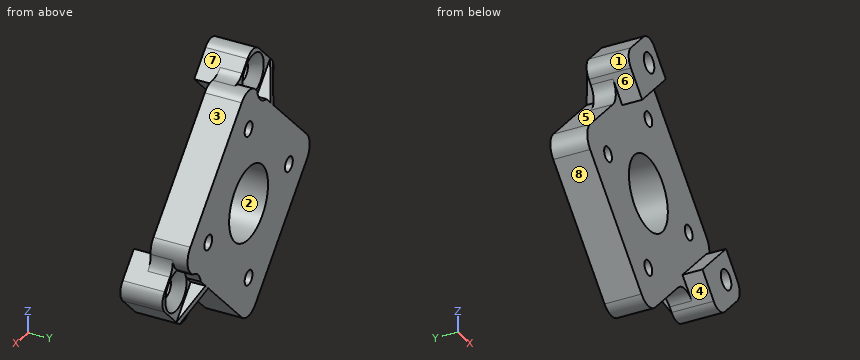
```python
from build123d import *

# Parameters (mm, degrees)
SKETCH1_R                                      = 0.5
SKETCH1_R_2                                    = 5
BOSS_EXTRUDE1_DEPTH                            = 5
SKETCH3_R                                      = 1.3
BOSS_EXTRUDE4_DEPTH                            = 5.7
BOSS_EXTRUDE6_DEPTH                            = 1
FILLET1_R                                      = 2.5
FILLET2_R                                      = 2
F_2_0MM_DOWEL_HOLE1_D                          = 2
F_2_0MM_DOWEL_HOLE1_DEPTH                      = 42.93
F_2_0MM_DOWEL_HOLE1_TIP                        = 0.600860619
SKETCH12_R                                     = 2.75
SKETCH12_R_2                                   = 2.625
CUT_EXTRUDE1_DEPTH                             = 10
CSK_FOR_M2_5_FLAT_HEAD_MACHINE_SCREW1_AT_COUNT = 2
CSK_FOR_M2_5_FLAT_HEAD_MACHINE_SCREW1_AT_PITCH = 28


with BuildPart() as part:
    # Sketch1 → Boss-Extrude1 (new body)
    with BuildSketch(Plane(origin=(0, 0, 0), x_dir=(1, 0, 0), z_dir=(0, 1, 0))):
        with BuildLine():
            Line((1.767766953, 14.961194078), (14.961194078, 1.767766953))
            ThreePointArc((14.961194078, 1.767766953), (15.693427125, 0), (14.961194078, -1.767766953))
            Line((14.961194078, -1.767766953), (1.767766953, -14.961194078))
            ThreePointArc((1.767766953, -14.961194078), (0, -15.693427125), (-1.767766953, -14.961194078))
            Line((-1.767766953, -14.961194078), (-14.961194078, -1.767766953))
            ThreePointArc((-14.961194078, -1.767766953), (-15.693427125, 0), (-14.961194078, 1.767766953))
            Line((-14.961194078, 1.767766953), (-1.767766953, 14.961194078))
            ThreePointArc((-1.767766953, 14.961194078), (0, 15.693427125), (1.767766953, 14.961194078))
        make_face()
        with Locations(Location((0, 10.365, 0), (0, 0, 270))):
            Circle(SKETCH1_R, mode=Mode.SUBTRACT)
        with Locations(Location((0, -10.365, 0), (0, 0, 270))):
            Circle(SKETCH1_R, mode=Mode.SUBTRACT)
        with Locations(Location((10.365, 0, 0), (0, 0, 270))):
            Circle(SKETCH1_R, mode=Mode.SUBTRACT)
        with Locations(Location((-10.365, 0, 0), (0, 0, 270))):
            Circle(SKETCH1_R, mode=Mode.SUBTRACT)
        with Locations(Location((0, 0, 0), (0, 0, 270))):
            Circle(SKETCH1_R_2, mode=Mode.SUBTRACT)
    extrude(amount=BOSS_EXTRUDE1_DEPTH)

    # Sketch3 → Boss-Extrude4 (add)
    # profile 1 of 4: a face of its own
    with BuildSketch(Plane(origin=(0, -2.7, 0), x_dir=(1, 0, 0), z_dir=(0, 1, 0))):
        Polygon((-4.949747468, -10.537489101), (-0.637994164, -14.849242405), (-4.949747468, -19.160995709), (-9.261500772, -14.849242405), align=None)
        with Locations(Location((-4.949747468, -14.849242405, 0), (0, 0, 90))):
            Circle(SKETCH3_R, mode=Mode.SUBTRACT)
    # profile 2 of 4: a face of its own
    with BuildSketch(Plane(origin=(0, -2.7, 0), x_dir=(1, 0, 0), z_dir=(0, 1, 0))):
        Polygon((-6.717514421, -8.769722148), (-11.029267725, -13.081475452), (-9.261500772, -14.849242405), (-4.949747468, -10.537489101), align=None)
    # profile 3 of 4: a face of its own
    with BuildSketch(Plane(origin=(0, -2.7, 0), x_dir=(1, 0, 0), z_dir=(0, 1, 0))):
        Polygon((19.160995709, 4.949747468), (14.849242405, 9.261500772), (10.537489101, 4.949747468), (14.849242405, 0.637994164), align=None)
        with Locations(Location((14.849242405, 4.949747468, 0), (0, 0, 90))):
            Circle(SKETCH3_R, mode=Mode.SUBTRACT)
    # profile 4 of 4: a face of its own
    with BuildSketch(Plane(origin=(0, -2.7, 0), x_dir=(1, 0, 0), z_dir=(0, 1, 0))):
        Polygon((13.081475452, 11.029267725), (14.849242405, 9.261500772), (10.537489101, 4.949747468), (8.769722148, 6.717514421), align=None)
    extrude(amount=BOSS_EXTRUDE4_DEPTH)


with BuildPart() as boss_extrude6_tool:
    # Sketch7 → Boss-Extrude6 (new body)
    with BuildSketch(Plane(origin=(2.707626069, -2.13e-07, 2.707626069), x_dir=(0.7071067811865474, 0, -0.7071067811865478), z_dir=(0.7071067811865467, -5.5755039757469385e-08, 0.7071067811865462))):
        Polygon((11.829161787, 5.00000052), (17.04887, 3.00000056), (11.829161787, 3.00000052), align=None)
        Polygon((-11.829161787, 5.00000052), (-17.04887, 3.00000056), (-11.829161787, 3.00000052), align=None)
    extrude(amount=-BOSS_EXTRUDE6_DEPTH)


with BuildPart() as part_1:
    add(part.part)


with BuildPart() as part_2:
    # Boss-Extrude6: joined with boss_extrude6_tool
    add(part_1.part.fuse(boss_extrude6_tool.part, tol=0.00001))

    # Fillet1
    fillet1_edges = [part_2.edges().sort_by_distance(p)[0] for p in [
        (-7.338376652, 1.5, 9.390584379),
        (-1.184018869, 1.5, 15.395267109),
        (9.390584379, 1.5, -7.338376652),
        (15.395267109, 1.5, -1.184018869),
    ]]
    fillet(fillet1_edges, radius=FILLET1_R)

    # Fillet2
    # the kernel refuses this fillet: 2 mm, written as the material it takes off along each edge
    with BuildSketch(Plane(origin=(-4.949747468, -7.7, 19.160995709), x_dir=(-0.7071067811865471, 0, -0.707106781186548), z_dir=(0, 1, 0)), Plane(origin=(13.081475452, -7.7, -11.029267725), x_dir=(0.7071067811865476, 0, 0.7071067811865476), z_dir=(0, 1, 0))) as fillet2_piece_1:
        with BuildLine():
            CenterArc((FILLET2_R, -FILLET2_R), FILLET2_R, 90, 90)
            Line((0, -FILLET2_R), (0, 0))
            Line((0, 0), (FILLET2_R, 0))
        make_face()
    extrude(amount=15.7, mode=Mode.SUBTRACT)
    with BuildSketch(Plane(origin=(-11.029267725, -7.7, 13.081475452), x_dir=(0.707106781186547, 0, 0.7071067811865479), z_dir=(0, 1, 0)), Plane(origin=(19.160995709, -7.7, -4.949747468), x_dir=(-0.7071067811865482, 0, -0.7071067811865469), z_dir=(0, 1, 0))) as fillet2_piece_2:
        with BuildLine():
            CenterArc((FILLET2_R, FILLET2_R), FILLET2_R, 180, 90)
            Line((0, FILLET2_R), (0, 0))
            Line((0, 0), (FILLET2_R, 0))
        make_face()
    extrude(amount=15.7, mode=Mode.SUBTRACT)

    # Ø2.0mm Dowel Hole1
    with Locations(Plane.XZ):
        with Locations((0, 10.365), (10.365, 0), (-10.365, 0), (0, -10.365)):
            Hole(F_2_0MM_DOWEL_HOLE1_D / 2, depth=F_2_0MM_DOWEL_HOLE1_DEPTH)
            with Locations((0, 0, -(F_2_0MM_DOWEL_HOLE1_DEPTH + F_2_0MM_DOWEL_HOLE1_TIP / 2))):  # 118° drill point
                Cone(0, F_2_0MM_DOWEL_HOLE1_D / 2, F_2_0MM_DOWEL_HOLE1_TIP, mode=Mode.SUBTRACT)

    # Sketch12 → Cut-Extrude1 (cut)
    with BuildSketch(Plane(origin=(0, 3, 0), x_dir=(1, 0, 0), z_dir=(0, 1, 0))):
        with Locations((-4.949747468, -14.849242405)):
            Circle(SKETCH12_R)
        with Locations((14.849242405, 4.949747468)):
            Circle(SKETCH12_R_2)
    extrude(amount=CUT_EXTRUDE1_DEPTH, mode=Mode.SUBTRACT)

    # Sketch13 → CSK for M2.5 Flat Head Machine Screw1 (revolve, cut)
    with BuildSketch(Plane(origin=(-4.949747468, 3, 14.849242405), x_dir=(0, 0, 1), z_dir=(1, 0, 0))):
        Polygon((0, 0), (0, 43.741161836), (1.35, 42.93), (1.35, 1.4), (2.75, 0), align=None)
    csk_for_m2_5_flat_head_machine_screw1 = revolve(axis=Axis((-4.949747468, 9.35, 14.849242405), (0, -1, 0)), mode=Mode.SUBTRACT)

    # CSK for M2.5 Flat Head Machine Screw1 at: CSK for M2.5 Flat Head Machine Screw1 ×2
    with Locations(*[Vector(0.7071067811865477, 0, -0.7071067811865475) * (i * CSK_FOR_M2_5_FLAT_HEAD_MACHINE_SCREW1_AT_PITCH) for i in range(1, CSK_FOR_M2_5_FLAT_HEAD_MACHINE_SCREW1_AT_COUNT)]):
        add(csk_for_m2_5_flat_head_machine_screw1, mode=Mode.SUBTRACT)


solid = part_2.part
```
For this review, take the finished solid that the model builds, in its own axes (mm). Face numbers are marked on the shaded views. A direction names the side the tool comes from. Give positions to 0.01 mm unless a question says otherwise; leave off trailing zeros. Write each loop counter-clockwise with the first axis right and the second up, starting at its lowest first coordinate (ties: lowest second). Pieces come first, ordered by that corner, then holes. Notation, with made-up numbers: M 21,78 L 62,78 A12 cw 62,85 Z; hole C 64,-16.75 d1. An arc over 180 degrees is marked long. Answer as CSV lines item,"result".
1. For the marked faces 4, 5, 6, 7 and 8, list the 3-axis set-ups (+Z, -Z, +X, -X, +Y, -Y) from which the entire face can be reached by the end or side of a thin tool; tool diameter is ignored.
Findings:
face 4,"-Z, -Y"
face 5,"-X, +Y"
face 6,"-X, -Y"
face 7,"+Z, +X, -Y"
face 8,"-Z, -X, +Y, -Y"
2. For pin 1 (4 mm diameter, centred on x = -5, z = -12, fed in from -Y); pin 2 (1.8 mm diameter, centred on x = 10.365, z = 0, fed in from -Y); pin 3 (4.5 mm diameter, centred on x = 14.85, z = -4.95, fed in from +Y); pin 4 (1.5 mm diameter, centred on x = -7, y = -1.5, fed in from -Z), all flat-tipped, find the tip position at first contact; note any pin that passes through.
Findings:
pin 1,"stops at y = 0"
pin 2,"passes through"
pin 3,"stops at y = 2.5"
pin 4,"stops at z = 8.77"
3. Consider section A-A, the plane y = -0.5. Write out the cut boundary in (x, z), then the cut area to 3 significant figures.
Findings:
outline,"M -9.62,11.67 L -6.72,8.77 L -0.64,14.85 L -3.54,17.75 A2 ccw -6.36,17.75 L -9.62,14.5 A2 ccw Z; M 8.77,-6.72 L 11.67,-9.62 A2 ccw 14.5,-9.62 L 17.75,-6.36 A2 ccw 17.75,-3.54 L 14.85,-0.64 Z; hole C -4.95,14.85 d2.7; hole C 14.85,-4.95 d2.7"
area,"90.0 mm2"
4. Wall thickness on line 1 (Y direction, x = 1.5, z = 9.5); line 2 (X direction, y = 1, z = 0.5); line 3 (X direction, y = 2.75, z = 4): over which ranges is each line inside the solid? List them lowest first.
Findings:
line 1,"y = 0 to 5"
line 2,"x = -15.64 to -11.23, -9.5 to -4.97, 4.97 to 9.5, 11.23 to 15.64"
line 3,"x = -12.73 to -3, 3 to 12.73"
5. Consider section D-D, the plane z = 5.5. Write out the cut boundary in (x, y), then the cut area to 3 significant figures.
Findings:
outline,"M -11.23,0 L 11.23,0 L 11.23,5 L -11.23,5 Z"
area,"112 mm2"
6. Draft analysis for pull direction X (two halves, no side actions). For the marked faces 1, 2 and 3, state which applies: +X half, -X half, draft (parallel to the pull), parting line (faces both ways), or undercut.
Findings:
face 1,"-X half"
face 2,"undercut"
face 3,"+X half"
7. Consider section B-B, the plane y = 4. Count the separate pieces of the cut face and the enclosed holes in it, then the cut area to 3 significant figures.
Findings:
separate pieces,"1"
enclosed holes,"5"
area,"466 mm2"
